Read the model definition and answer for the solid it produces. Units are mm, in the model's axes. A direction names the side the tool comes from. Round coordinates to 2 decimals unless told otherwise and drop trailing zeros. Loops run counter-clockwise (first coordinate to the right, second up) from the corner with the lowest first, then second, coordinate; pieces in that order, holes last. Notation, with made-up numbers: (59, -4) - (102, -4) arc R25 ccw to (102, 21) - close; hole circle Ø5 at (-21, 71). An arc over 180 degrees is marked (long way). Use CSV: the item, a comma, the result in double quotes. Start each with the question number.
1. Consider line 1 along Y through (x, z) = (15, -4); line 2 along Z through (x, y) = (-41, -5); line 3 along Z through (x, y) = (-10, -9). Determine where each line is inside the solid, lowest interval first.
2. Find section B-B (x = -32). Give the vertices of the cut face in (y, z).
3. Find section D-D (y = 0). Give the vertices of the cut face in (x, z), and give its area (3 significant figures).
4. Determine the mould class of faces 1 (the flat face through (12.161, 26.853, 2.283)), 2 (the flat face through (-44.466, 0, 3)), 3 (the flat face through (-4, 0, -29.5)), 4 (the flat face through (-14.44, -0.2, -11.32)) for opening direction Z: +Z half, -Z half, draft (parallel to the pull), parting line (faces both ways), or undercut.
5. Find section C-C (z = 18). Give the vertices of the cut face in (x, y), and give its area (3 significant figures).
6. A tool of negligible diameter and unlimited length cuts with its end or side. For faces 5 (the flat face through (-0.6, 21.844, 12.4)), 6 (the flat face through (-30, -5, 29.788)), 7 (the flat face through (-15, -32.004, -6)), from which of +Z, -Z, +X, -X, +Y, -Y can it reach the whole face along a straight path? Write none if from no direction.
7. Find section A-A (y = 11). Give the vertices of the cut face in (x, z).
8. Given pin 1 Ø8 at (y, z) = (19.5, -6) entering from +X; pin 2 Ø1.5 at (x, y) = (-20.5, -6) entering from +Z; pin 3 Ø4 at (x, z) = (7.5, 6) entering from -Y, each flat-ended and moving along its own axis, determine where each tip first touches the part or whether it passes through.
from build123d import *

# Parameters (mm, degrees)
F1_DEPTH = 32.004
F2_DEPTH = 32.004
F4_DEPTH = 53.848
F5_R     = 13.9464432641
F6_DEPTH = 25.4


with BuildPart() as f1:
    # F0 (on Front) → F1 (new body)
    with BuildSketch(Plane.XZ):
        Polygon((-13.9585789293, 34.9684022367), (-44.4659888744, 34.6805937588), (-44.4659888744, -29.5000895858), (37.5586524606, -29.5000895858), align=None)
    extrude(amount=F1_DEPTH)

    # F2 (add): a face of the model
    f2_faces = [f1.faces().sort_by_distance(p)[0] for p in [
        (-14.3434422771, 0, -2.2296991065),
    ]]
    extrude(f2_faces, amount=F2_DEPTH)

    # F3 (on face) → F4 (cut)
    with BuildSketch(Plane.XZ.offset(32.004)):
        Polygon((-44.4659888744, 34.6805937588), (-44.4659888744, 29.7878943384), (-14.8219969124, 29.7878943384), (32.6659567654, -29.5000895858), (37.5586524606, -29.5000895858), (-13.9585789293, 34.9684022367), align=None)
    extrude(amount=-F4_DEPTH, mode=Mode.SUBTRACT)

    # F5 (on face) → F6 (cut)
    with BuildSketch(Plane(origin=(5.5052949063, 0, 4.409581372), x_dir=(0, 1, 0), z_dir=(0.7804989961, 0, 0.6251570339))):
        Circle(F5_R)
    extrude(amount=-F6_DEPTH, mode=Mode.SUBTRACT)


solid = f1.part
Filled sheet:
1,line 1,"y = 21.84 to 32"
1,line 2,"z = -29.5 to 29.79"
1,line 3,"z = -29.5 to -16.86, 5.64 to 23.77"
2,outline,"(-32, -29.5) - (32, -29.5) - (32, 34.8) - (21.84, 34.8) - (21.84, 29.79) - (-32, 29.79) - close"
3,outline,"(-44.47, -29.5) - (32.67, -29.5) - (14.22, -6.48) - (-5.6, -22.35) - (-23.04, -0.58) - (-3.21, 15.29) - (-14.82, 29.79) - (-44.47, 29.79) - close"
3,area,"2,460 mm²"
4,face 1,"+Z half"
4,face 2,"draft"
4,face 3,"-Z half"
4,face 4,"undercut"
5,outline,"(-44.47, -32) - (-5.38, -32) - (-5.38, 21.84) - (-0.4, 21.84) - (-0.4, 32) - (-44.47, 32) - close"
5,area,"2,550 mm²"
6,face 5,"+Z, +X, -Y"
6,face 6,"+Z, +X, -X, -Y"
6,face 7,"+Z, -Z, +X, -X, -Y"
7,outline,"(-44.47, -29.5) - (32.67, -29.5) - (10.87, -2.28) - (-8.96, -18.16) - (-19.68, -4.78) - (0.15, 11.1) - (-14.82, 29.79) - (-44.47, 29.79) - close"
8,pin 1,"stops at x = 21.37"
8,pin 2,"stops at z = 29.79"
8,pin 3,"stops at y = 21.84"
